Work out the finished part from the listing and answer in its coordinate system (mm). A direction names the side the tool comes from. Round coordinates to 2 decimals unless told otherwise and drop trailing zeros. Loops run counter-clockwise (first coordinate to the right, second up) from the corner with the lowest first, then second, coordinate; pieces in that order, holes last. Notation, with made-up numbers: (72, -21) - (111, -21) arc R26 cw to (111, 0) - close; hole circle Ø8 at (79, 40). An arc over 180 degrees is marked (long way). Answer as CSV lines item,"result". Start each with the question number.
Q1. Section B-B on y = 0 is taken. Write down the section's boundary in (x, z), then the cut area to 3 significant figures.
Q2. Section A-A on x = 0 is taken. Write down the section's boundary in (y, z).
Q3. For faces 1 (the face through (-0.05, -1.5, -4.93)), 2 (the face through (0, -5, 11)), 3 (the face through (0, 1.264, -5)), determine the directions among +Z, -Z, +X, -X, +Y, -Y from which every point of the face is accessible in a straight line to the end or side of a thin tool.
Q4. Section D-D on y = -3.25 is taken. Write down the section's boundary in (x, z), then the cut area to 3 significant figures.
Q5. Each of these flat-tipped pins is pushed along its axis until it touches: pin 1 Ø0.8 at (x, z) = (0, -5.5) entering from +Y; pin 2 Ø2 at (y, z) = (-0.5, -6.5) entering from -X; pin 3 Ø1.5 at (y, z) = (-2.5, -5) entering from +X. Where does it stop, or does it pass through?
Q6. Straight lines are drawn through the part: L1, parallel to Z at x = -5, y = 2.5; L2, parallel to Y at x = 0, z = -2; L3, parallel to Y at x = -5.5, z = 20.5. For each, find the intervals that lie inside material, in ascending order. Write a range as [from, to].
Q7. Section C-C on z = -2.5 is taken. Write down the section's boundary in (x, y).
```python
from build123d import *

# Parameters (mm, degrees)
SKETCH_1_W          = 12
SKETCH_1_H          = 10
EXTRUDE_1_DEPTH     = 22.4
SKETCH_2_R          = 1.5
EXTRUDE_2_DEPTH     = 10
FILLET_1_R          = 1
FILLET_2_R          = 1
CUT_EXTRUDE_1_DEPTH = 10


with BuildPart() as part:
    # ｽｹｯﾁ1 → ﾎﾞｽ - 押し出し1 (new body)
    with BuildSketch(Plane.XY):
        Rectangle(SKETCH_1_W, SKETCH_1_H)
    extrude(amount=EXTRUDE_1_DEPTH)

    # ｽｹｯﾁ2 → ﾎﾞｽ - 押し出し2 (add)
    with BuildSketch(Plane.XY):
        Circle(SKETCH_2_R)
    extrude(amount=-EXTRUDE_2_DEPTH)

    # ﾌｨﾚｯﾄ1
    fillet_1_edges = [part.edges().sort_by_distance(p)[0] for p in [
        (-6, 5, 11.2),
    ]]
    fillet(fillet_1_edges, radius=FILLET_1_R)

    # ﾌｨﾚｯﾄ2
    fillet_2_edges = [part.edges().sort_by_distance(p)[0] for p in [
        (-6, -5, 11.2),
        (6, 5, 11.2),
        (6, -5, 11.2),
    ]]
    fillet(fillet_2_edges, radius=FILLET_2_R)

    # ｽｹｯﾁ3 → ｶｯﾄ - 押し出し1 (cut)
    with BuildSketch(Plane.XY):
        Polygon((0, 1.5), (-1.572523441, 1.5), (-1.572523441, 1.264308846), (1.824127191, 1.264308846), (1.824127191, 1.5), align=None)
    extrude(amount=-CUT_EXTRUDE_1_DEPTH, mode=Mode.SUBTRACT)


solid = part.part
```
Findings:
1,outline,"(-6, 0) - (-1.5, 0) - (-1.5, -10) - (1.5, -10) - (1.5, 0) - (6, 0) - (6, 22.4) - (-6, 22.4) - close"
1,area,"299 mm^2"
2,outline,"(-5, 0) - (-1.5, 0) - (-1.5, -10) - (1.26, -10) - (1.26, 0) - (5, 0) - (5, 22.4) - (-5, 22.4) - close"
3,face 1,"-Z"
3,face 2,"+Z, -Z, +X, -X, -Y"
3,face 3,"-Z, +X, -X, +Y"
4,outline,"(-6, 0) - (6, 0) - (6, 22.4) - (-6, 22.4) - close"
4,area,"269 mm^2"
5,pin 1,"stops at y = 1.26"
5,pin 2,"stops at x = -1.5"
5,pin 3,"passes through"
6,L1,"z = [0, 22.4]"
6,L2,"y = [-1.5, 1.26]"
6,L3,"y = [-4.87, 4.87]"
7,outline,"(-0.81, 1.26) arc R1.5 ccw (long way) to (0.81, 1.26) - close"
